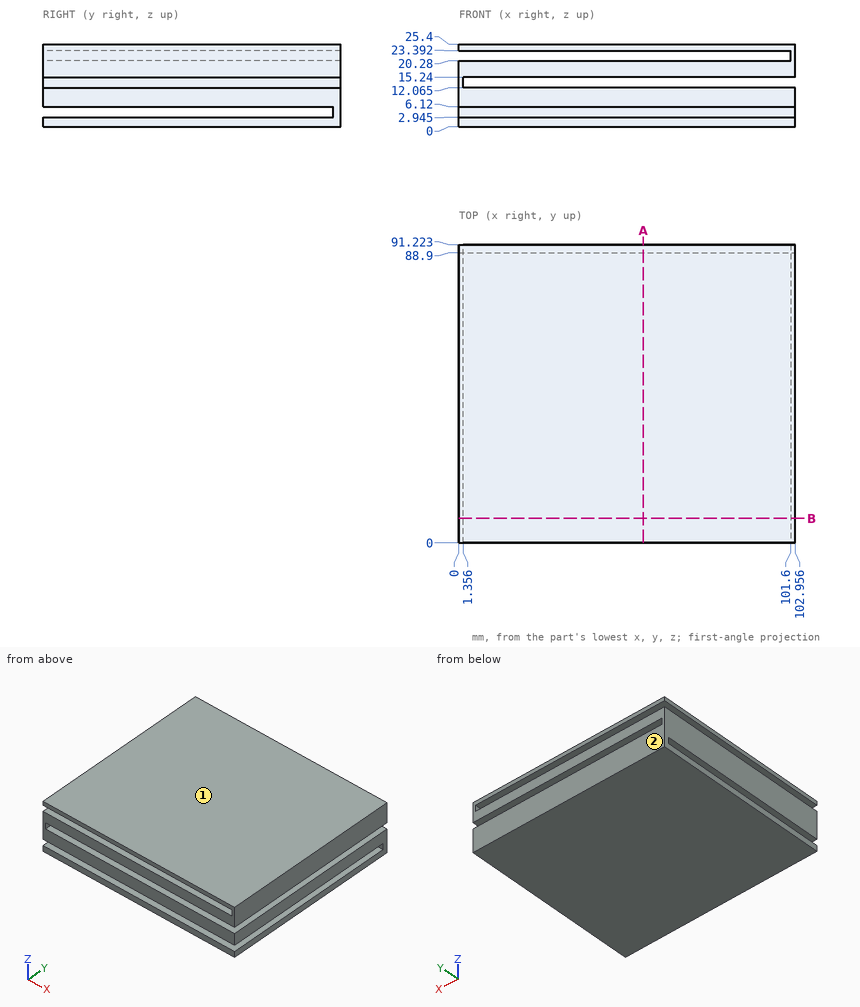
Geometry check sheet. Reference: drawing and pictorial views, mm from the part's lowest x, y, z. Give positions to 0.01 mm unless a question says otherwise; leave off trailing zeros. Order: outer loops, then holes, each group sorted by start corner. A loop starts at its lowest first (then second) coordinate and runs counter-clockwise, first axis right, second up. Notation, with made-up numbers: M 84.5,86 L 121.5,86 A17 ccw 121.5,102 Z; hole C 15.5,61.5 d11. An arc over 180 degrees is marked long. Answer in a Markdown table with one row per item.
1) Gauge pin test, flat end, axial feed: P1, Ø1, axis at x = 81.5, z = 5, coming from the -Y side. Record the tip position at first contact, or that the pin passes through.
Filled sheet:
| item | result |
|---|---|
| P1 | stops at y = 88.9 |
2) Cross-section at A-A, the plane x = 56.5. Enter the section's corners in (y, z) (1 decimal).
Filled sheet:
| item | result |
|---|---|
| outline | M 0,0 L 91.2,0 L 91.2,12.1 L 0,12.1 L 0,6.1 L 88.9,6.1 L 88.9,2.9 L 0,2.9 Z; M 0,15.2 L 91.2,15.2 L 91.2,20.3 L 0,20.3 Z; M 0,23.4 L 91.2,23.4 L 91.2,25.4 L 0,25.4 Z |
3) Thickness scan on L1, parallel to Z at x = 63, y = 82 (1 decimal); L2, parallel to X at y = 84.5, z = 20.5 (1 decimal); L3, parallel to Y at x = 92, z = 5.5. Record the ranges inside material, lowest first. Write a range as [from, to].
Filled sheet:
| item | result |
|---|---|
| L1 | z = [0, 2.9], [6.1, 12.1], [15.2, 20.3], [23.4, 25.4] |
| L2 | x = [101.6, 103] |
| L3 | y = [88.9, 91.22] |
4) Cross-section at B-B, the plane y = 7.5. Enter the section's corners in (x, z) (1 decimal).
Filled sheet:
| item | result |
|---|---|
| outline | M 0,0 L 103,0 L 103,2.9 L 0,2.9 Z; M 0,6.1 L 103,6.1 L 103,12.1 L 1.4,12.1 L 1.4,15.2 L 103,15.2 L 103,25.4 L 0,25.4 L 0,23.4 L 101.6,23.4 L 101.6,20.3 L 0,20.3 Z |
5) Release check for a two-part mould opening along Y. For the marked faces 1 and 2 record: +Y half, -Y half, draft (parallel to the pull), parting line (faces both ways), or undercut.
Filled sheet:
| item | result |
|---|---|
| face 1 | draft |
| face 2 | +Y half |
